from build123d import *

# Parameters (mm, degrees)
EXTRUDE_1_DEPTH     = 56.5
CUT_EXTRUDE_1_REACH = 61.662
SKETCH_2_W          = 20
SKETCH_2_H          = 20
CUT_EXTRUDE_2_DEPTH = 60.661545404
EXTRUDE_2_DEPTH     = 46


with BuildPart() as part:
    # 草图1 → 凸台-拉伸1 (new body)
    with BuildSketch(Plane.XY):
        Polygon((-16.5, 0), (-16.5, 1.5), (-14, 1.5), (-14, 5), (16, 5), (16, 1.5), (18.5, 1.5), (18.5, 0), (14, 0), (14, 3), (-12, 3), (-12, 0), align=None)
    extrude(amount=EXTRUDE_1_DEPTH)

    # 草图2 → 切除-拉伸1 (cut, up to next)
    with BuildSketch(Plane(origin=(0, 5, 0), x_dir=(1, 0, 0), z_dir=(0, 1, 0)), mode=Mode.PRIVATE) as cut_extrude_1_sk1:
        with Locations((1, -46.5)):
            Rectangle(SKETCH_2_W, SKETCH_2_H)
    cut_extrude_1_tool1 = extrude(cut_extrude_1_sk1.sketch, amount=-CUT_EXTRUDE_1_REACH, mode=Mode.PRIVATE) & part.part
    add(cut_extrude_1_tool1.solids().sort_by_distance((1, 5, 46.5))[0], mode=Mode.SUBTRACT)

    # 草图3 → 切除-拉伸2 (cut, through all)
    with BuildSketch(Plane.XY.offset(56.5)):
        Polygon((-16.3, 0), (-16.3, 1.3), (-13.8, 1.3), (-13.8, 4.8), (15.8, 4.8), (15.8, 1.3), (18.3, 1.3), (18.3, 0), (18.5, 0), (18.5, 1.5), (16, 1.5), (16, 5), (-14, 5), (-14, 1.5), (-16.5, 1.5), (-16.5, 0), align=None)
    extrude(amount=-CUT_EXTRUDE_2_DEPTH, mode=Mode.SUBTRACT)

    # 草图4 → 凸台-拉伸2 (add)
    with BuildSketch(Plane(origin=(0, 0, 0), x_dir=(-1, 0, 0), z_dir=(0, 0, -1))):
        Polygon((-15.8, 1.3), (-18.3, 1.3), (-18.3, 0), (-14, 0), (-14, 3), (12, 3), (12, 0), (16.3, 0), (16.3, 1.3), (13.8, 1.3), (13.8, 4.8), (-15.8, 4.8), align=None)
    extrude(amount=EXTRUDE_2_DEPTH)


solid = part.part
CAD build for the part. Positions are in the model's coordinates, mm. A direction names the side the tool comes from. Give positions to 0.01 mm unless a question says otherwise; leave off trailing zeros. Order: outer loops, then holes, each group sorted by start corner. A loop starts at its lowest first (then second) coordinate and runs counter-clockwise, first axis right, second up. Notation, with made-up numbers: (-12.75, 43.5) - (40.25, 43.5) arc R9 ccw to (40.25, 56.5) - close; hole circle Ø10 at (0, 40.5). An arc over 180 degrees is marked (long way). Answer in a Markdown table with one row per item.
1. Probe probe 1 along X at (y, z) = (2.3, -1); probe 2 along X at (y, z) = (3.55, 39); probe 3 along Z at (x, y) = (-2, 3.9). List the from-to ranges inside material, lowest first. Write a range as [from, to].
Data:
| item | result |
|---|---|
| probe 1 | x = [-13.8, -12], [14, 15.8] |
| probe 2 | x = [-13.8, -9], [11, 15.8] |
| probe 3 | z = [-46, 36.5] |
2. Flat gauge pins, fed straight in: pin 1 (2.5 mm diameter, centred on y = 1.5, z = -14.5, fed in from -X); pin 2 (2 mm diameter, centred on x = 0.5, y = 3.5, fed in from +Z); pin 3 (2 mm diameter, centred on y = 2.5, z = 24.5, fed in from +X); pin 4 (2 mm diameter, centred on y = 3.5, z = 44.5, fed in from -X). Where does each tip first touch, or does it go through?
Data:
| item | result |
|---|---|
| pin 1 | stops at x = -16.3 |
| pin 2 | stops at z = 36.5 |
| pin 3 | stops at x = 15.8 |
| pin 4 | stops at x = -13.8 |
3. Saw through at D-D, the plane x = 12.5. Give the cut face in (y, z).
Data:
| item | result |
|---|---|
| outline | (3, -46) - (4.8, -46) - (4.8, 56.5) - (3, 56.5) - close |
4. Saw through at C-C, the plane z = 10. Give the cut face in (x, y).
Data:
| item | result |
|---|---|
| outline | (-16.3, 0) - (-12, 0) - (-12, 3) - (14, 3) - (14, 0) - (18.3, 0) - (18.3, 1.3) - (15.8, 1.3) - (15.8, 4.8) - (-13.8, 4.8) - (-13.8, 1.3) - (-16.3, 1.3) - close |
5. Saw through at A-A, the plane z = 41.5. Give the cut face in (x, y), plus the area to 3 significant figures.
Data:
| item | result |
|---|---|
| outline | (-16.3, 0) - (-12, 0) - (-12, 3) - (-9, 3) - (-9, 4.8) - (-13.8, 4.8) - (-13.8, 1.3) - (-16.3, 1.3) - close; (11, 3) - (14, 3) - (14, 0) - (18.3, 0) - (18.3, 1.3) - (15.8, 1.3) - (15.8, 4.8) - (11, 4.8) - close |
| area | 34.6 mm² |
6. Pull direction X, two halves, no side cores. Call faces 4 (the flat face through (14, 1, 6)), 5 (the flat face through (15.8, 3, 6)), 6 (the flat face through (-12, 2, 6)), 7 (the flat face through (-15, 1.3, 6)): pulls with the +X half, pulls with the -X half, needs draft (parallel to the pull), parting line crosses it, or undercut.
Data:
| item | result |
|---|---|
| face 4 | undercut |
| face 5 | pulls with the +X half |
| face 6 | undercut |
| face 7 | needs draft |
7. Saw through at B-B, the plane y = 3.8. Give the cut face in (x, z), plus the area to 3 significant figures.
Data:
| item | result |
|---|---|
| outline | (-13.8, -46) - (15.8, -46) - (15.8, 56.5) - (11, 56.5) - (11, 36.5) - (-9, 36.5) - (-9, 56.5) - (-13.8, 56.5) - close |
| area | 2,630 mm² |
8. Tool access for faces 1 (the flat face through (1, 4, 36.5)), 2 (the flat face through (1, 3, -5)), 3 (the flat face through (-13.8, 3, 6)): list every direction of +Z, -Z, +X, -X, +Y, -Y with a clear straight run to the whole face (end or side of a thin tool).
Data:
| item | result |
|---|---|
| face 1 | +Z, +Y, -Y |
| face 2 | +Z, -Z, -Y |
| face 3 | +Z, -Z, -X, +Y |
